Design review of the part built by this model. Coordinates are the model's own, in mm. A direction names the side the tool comes from. Round coordinates to 2 decimals unless told otherwise and drop trailing zeros. Write each loop counter-clockwise with the first axis right and the second up, starting at its lowest first coordinate (ties: lowest second). Pieces come first, ordered by that corner, then holes. Notation, with made-up numbers: (25.5, -15.5) - (44.5, -15.5) arc R17 cw to (44.5, 12.5) - close; hole circle Ø9 at (12, 76.5). An arc over 180 degrees is marked (long way). Use one line per item in the form item = value.
Autodesk Inventor part; units mm, degrees
ref_plane "Work Plane1" through (0, 0, 20) normal (0, 0, 1) x (1, 0, 0)
ref_plane "YZ Plane" through (0, 0, 0) normal (1, 0, 0) x (0, 1, 0)
ref_plane "XZ Plane" through (0, 0, 0) normal (0, 1, 0) x (-1, 0, 0)
sketch "Sketch1" plane through (0, 0, 0) normal (0, 0, 1) x (1, 0, 0)
  line L0 (-6, 11.5) -> (6, 11.5)
  line L1 (6, 11.5) -> (6, -11.5)
  line L2 (6, -11.5) -> (-6, -11.5)
  line L3 (-6, -11.5) -> (-6, 11.5)
  line L4 (0, 0) -> (0, -6.2119)
  line L5 (0, 0) -> (2.7529, 0)
  dimension "d0" = 12
  dimension "d1" = 23
extrude "Extrusion1" add sketch "Sketch1" along normal blind 22
ref_plane "Work Plane1" through (0, 0, 20) normal (0, 0, 1) x (1, 0, 0)
sketch "Sketch2" plane through (0, 0, 20) normal (0, 0, 1) x (1, 0, 0)
  line L0 (6, 11.5) -> (-6, 11.5)
  line L1 (-6, 11.5) -> (6, 11.5)
  line L2 (6, 11.5) -> (6, 16)
  line L3 (6, 16) -> (-6, 16)
  line L4 (-6, 16) -> (-6, 11.5)
  line L5 (6, -11.5) -> (6, 11.5)
  point P0 (0, 0)
  dimension "d5" = 4.5
extrude "Extrusion2" add sketch "Sketch2" against normal blind 2
sketch "Sketch3" plane through (0, 0, 20) normal (0, 0, 1) x (1, 0, 0)
  circle A0 centre (0, 14.5) radius 1
  line L0 (6, 16) -> (-6, 16)
  point P0 (0, 0)
  dimension "d8" = 2
  dimension "d9" = 1.5
extrude "Extrusion3" cut sketch "Sketch3" against normal blind 2
fillet "Fillet1" radius 1 6 edges at (6, 16, 19) (-6, 16, 19) (6, 11.5, 9) (6, 11.5, 21) (-6, 11.5, 21) (-6, 11.5, 9)
mirror "Mirror1" about plane through (0, 0, 0) normal (0, 1, 0) of "Extrusion2", "Extrusion3", "Fillet1"
fillet_without_effect "Fillet2"
sketch "Sketch4" plane through (0, 0, 22) normal (0, 0, 1) x (1, 0, 0)
  circle A0 centre (0, 5.5) radius 6
  line L0 (5, 11.5) -> (-5, 11.5)
  point P0 (0, 0)
  dimension "d14" = 12
extrude "Extrusion4" add sketch "Sketch4" along normal blind 5
properties part number "MicroServo"
Q1. We need section B-B on z = 19.5. Write out the cut boundary in (x, y), then the cut area to 3 significant figures.
Calculated:
outline = (-6, -15) arc R1 ccw to (-5, -16) - (5, -16) arc R1 ccw to (6, -15) - (6, 15) arc R1 ccw to (5, 16) - (-5, 16) arc R1 ccw to (-6, 15) - close; hole circle Ø2 at (0, -14.5); hole circle Ø2 at (0, 14.5)
area = 377 mm2
Q2. For P1, Ø1.5, axis at x = 1.5, z = 22.5, coming from the -Y side; P2, Ø4.5, axis at x = 0, y = 14.5, coming from the +Z side; P3, Ø4.5, axis at x = 3, y = -14.5, coming from the -Z side; P4, Ø1.8, axis at x = 0, y = 14.5, coming from the +Z side, all flat-tipped, find the tip position at first contact; note any pin that passes through.
Calculated:
P1 = -11.5
P2 = 20
P3 = 18
P4 = through
Q3. Draft analysis for pull direction Y (two halves, no side actions). For faces 1 (the cylindrical face through (-0.217, 13.524, 19.014)), 2 (the flat face through (0, 0, 0)), 3 (the cylindrical face through (-5.715, -11.199, 21.014)), 4 (the cylindrical face through (5.699, 15.715, 18.986)), state which applies: released by +Y, released by -Y, zero draft, split by the parting line, or undercut.
Calculated:
face_1 = undercut
face_2 = zero draft
face_3 = released by -Y
face_4 = released by +Y
Q4. We need section C-C on x = -3.5. Write out the cut boundary in (y, z), then the cut area to 3 significant figures.
Calculated:
outline = (-16, 18) - (-11.5, 18) - (-11.5, 0) - (11.5, 0) - (11.5, 18) - (16, 18) - (16, 20) - (11.5, 20) - (11.5, 22) - (10.37, 22) - (10.37, 27) - (0.63, 27) - (0.63, 22) - (-11.5, 22) - (-11.5, 20) - (-16, 20) - close
area = 573 mm2
Q5. We need section A-A on y = -14.5. Write out the cut boundary in (x, z).
Calculated:
outline = (-6, 18) - (-1, 18) - (-1, 20) - (-6, 20) - close; (1, 18) - (6, 18) - (6, 20) - (1, 20) - close
Q6. We need section D-D on z = 12.25. Write out the cut boundary in (x, y).
Calculated:
outline = (-6, -10.5) arc R1 ccw to (-5, -11.5) - (5, -11.5) arc R1 ccw to (6, -10.5) - (6, 10.5) arc R1 ccw to (5, 11.5) - (-5, 11.5) arc R1 ccw to (-6, 10.5) - close
Q7. Machinability: for faces 5 (the flat face through (0, 11.5, 9)), 6 (the cylindrical face through (-1.301, 11.357, 24.465)), 7 (the cylindrical face through (5.699, -11.215, 21.014)), 8 (the cylindrical face through (5.715, 11.199, 9.126)), which of the approach directions +Z, -Z, +X, -X, +Y, -Y give a long, thin tool a straight path to every point of the face, cutting with its end or side? Answer none if there is none.
Calculated:
face_5 = -Z, +X, -X, +Y
face_6 = +Z
face_7 = +Z, +X, -Y
face_8 = -Z, +X, +Y
Q8. To check wall thickness, follow line 1 along Y through (x, z) = (0, 18.5); line 2 along X through (y, z) = (-14.5, 19.2); line 3 along Z through (x, y) = (-4, -12). State the ranges of each line that lie inside material, in increasing order. Write a range as from..to.
Calculated:
line_1 = -16..-15.5, -13.5..13.5, 15.5..16
line_2 = -6..-1, 1..6
line_3 = 18..20
